from build123d import *

# Parameters (mm, degrees)
F0_R     = 150
F1_DEPTH = 10


# Not quite as in the source:
# - a fillet or chamfer that OpenCascade refuses, or shapes differently, is made with other operations: its cross-section is extruded or revolved along the edge and cut away or added


with BuildPart() as f1:
    # F0 (on Top) → F1 (new body)
    with BuildSketch(Plane.XY):
        Circle(F0_R)
    extrude(amount=F1_DEPTH)

    # F2 (on Front) → F3 (revolve)
    with BuildSketch(Plane.XZ):
        with BuildLine():
            Line((130.4040820577, 5), (150, 5))
            ThreePointArc((150, 5), (140.2020410289, 13), (130.4040820577, 5))
        make_face()
    revolve(axis=Axis((0, 0, 19.3104613572), (0, 0, 1)))

    # F4: fillet of radius 3 on 4 edges, made by hand

    # F4_s1 → F4_t2 (revolve)
    with BuildSketch(Plane.XZ):
        with BuildLine():
            ThreePointArc((133.8123303651, 10.6923076923), (132.9144664967, 10.1783801706), (131.8954171659, 10))
            Line((131.8954171659, 10), (133.0606126003, 10))
            ThreePointArc((133.0606126003, 10), (133.4276219564, 10.3557627905), (133.8123303651, 10.6923076923))
        make_face()
    revolve(axis=Axis((0, 0, 10), (0, 0, 1)))

    # F4_s3 → F4_t4 (revolve, cut)
    with BuildSketch(Plane.XZ):
        with BuildLine():
            ThreePointArc((150, 3), (149.1213203436, 0.8786796564), (147, 0))
            Line((147, 0), (150, 0))
            Line((150, 0), (150, 3))
        make_face()
    revolve(axis=Axis((0, 0, 0), (0, 0, 1)), mode=Mode.SUBTRACT)

    # F4_s5 → F4_t6 (revolve, cut)
    with BuildSketch(Plane.XZ):
        with BuildLine():
            ThreePointArc((150, 7.0197267354), (149.2394651563, 9.01592207), (147.3434694574, 10))
            Line((147.3434694574, 10), (150, 10))
            Line((150, 10), (150, 7.0197267354))
        make_face()
    revolve(axis=Axis((0, 0, 10), (0, 0, 1)), mode=Mode.SUBTRACT)


solid = f1.part
Design review of the part built by this model. Coordinates are the model's own, in mm. Give positions to 0.01 mm unless a question says otherwise; leave off trailing zeros. Loops run counter-clockwise (first coordinate to the right, second up) from the corner with the lowest first, then second, coordinate; pieces in that order, holes last. Notation, with made-up numbers: M 18.25,-28 L 41.25,-28 A25 cw 41.25,-8 Z; hole C 68,-17 d3. An arc over 180 degrees is marked long. One line per question, with ' | ' between items. Start each with the question number.
1. Insertion check: P1, Ø2, axis at x = -56.5, y = 114.5, coming from the +Z side; P2, Ø6, axis at x = -27, z = 5, coming from the -Y side; P3, Ø5, axis at y = -58, z = 5, coming from the -X side. Each pin has a flat end and moves straight along its axis. Give the tip position at first contact, or say it passes through.
2. To check wall thickness, follow L1, parallel to Z at x = 58, y = 2.5; L2, parallel to X at y = -4, z = 11; L3, parallel to Y at x = -71.5, z = 7.5. State the ranges of each line that lie inside material, in increasing order.
3. The part is to be moulded in two halves that separate along X. For faces 1 (the face through (-2, 2, 0)), 2 (the face through (-19.527, 148.724, 4.982)), 3 (the face through (-2, 2, 10)), say which applies: released by +X, released by -X, zero draft, split by the parting line, or undercut.
4. Add section A-A (y = 0). Write out the cut boundary in (x, z).
Worked out:
1) P1: stops at z = 10 | P2: stops at y = -148.07 | P3: stops at x = -139.35
2) L1: z = 0 to 10 | L2: x = -146.15 to -134.14, 134.14 to 146.15 | L3: y = -131.82 to 131.82
3) face 1: zero draft | face 2: split by the parting line | face 3: undercut
4) outline: M -150,3 A3 ccw -147,0 L 147,0 A3 ccw 150,3 L 150,7.02 A3 ccw 147.34,10 A10 ccw 133.81,10.69 A3 cw 131.9,10 L -131.9,10 A3 cw -133.81,10.69 A10 ccw -147.34,10 A3 ccw -150,7.02 Z
